Can you work these out from the drawing? Everything is in mm from the part's minimum corner. A direction names the side the tool comes from. Round coordinates to 2 decimals unless told otherwise and drop trailing zeros. Write each loop counter-clockwise with the first axis right and the second up, starting at its lowest first coordinate (ties: lowest second). Pieces come first, ordered by that corner, then holes. Notation, with made-up numbers: (36.5, 27.25) - (46.5, 27.25) arc R17 ccw to (46.5, 54.25) - close; hole circle Ø8 at (11, 66). An arc over 180 degrees is marked (long way). One line per item, written item: value. Start each with the question number.
Item 1: If I drill on line 1 (Y direction, x = 5, z = 16); line 2 (Y direction, x = 4, z = 15); line 3 (Z direction, x = 27.5, y = 13), over which ranges is the centre line in solid material (lowest first)?
Item 2: Imagine slicing it at D-D, the plane y = 16.5. Please give me the cut outline in (x, z), then the cut area to 3 significant figures.
Item 3: Imagine slicing it at B-B, the plane z = 26.67. Please give me the cut outline in (x, y), then the cut area to 3 significant figures.
Item 4: For the marked faces 1 and 2, which set-ups out of +Z, -Z, +X, -X, +Y, -Y let a thin tool reach every point of the face, with its end or its side?
Item 5: For P1, Ø8, axis at x = 20.5, z = 39.5, coming from the +Y side; P2, Ø4, axis at y = 14, z = 27, coming from the -X side, each with a flat end and sliding along its axis, tell me the tip position at first contact or that it passes through.
Item 6: Imagine slicing it at A-A, the plane x = 26.67. Please give me the cut outline in (y, z).
Item 7: Imagine slicing it at C-C, the plane y = 28.5. Please give me the cut outline in (x, z).
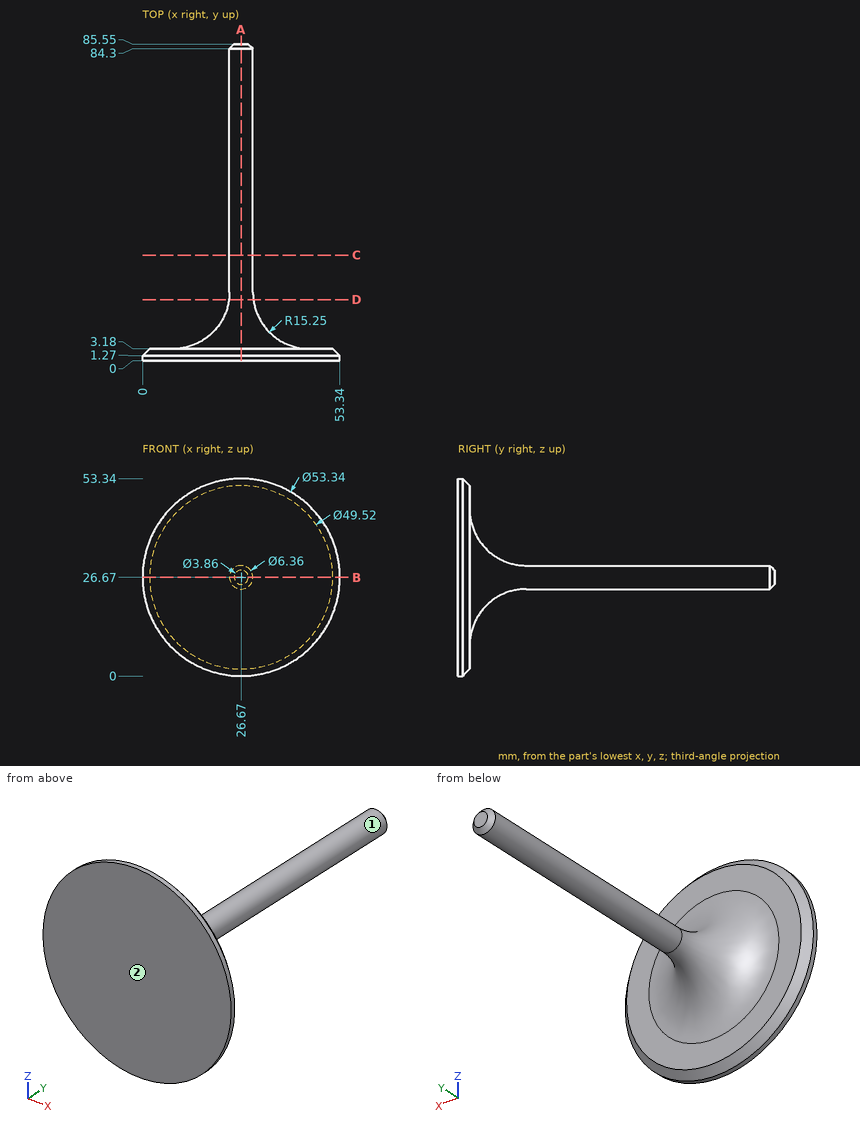
Values follow:
1. line 1: y = 0 to 3.18
1. line 2: y = 0 to 2.44
1. line 3: z = 22.57 to 30.77
2. outline: circle Ø6.61 at (26.67, 26.67)
2. area: 34.3 mm^2
3. outline: (0, 0) - (53.34, 0) - (53.34, 1.27) - (51.43, 3.18) - (45.1, 3.18) arc R15.25 cw to (29.85, 18.43) - (29.85, 84.3) - (28.6, 85.55) - (24.74, 85.55) - (23.49, 84.3) - (23.49, 18.43) arc R15.25 cw to (8.24, 3.18) - (1.91, 3.18) - (0, 1.27) - close
3. area: 788 mm^2
4. face 1: +Y
4. face 2: +Z, -Z, +X, -X, -Y
5. P1: stops at y = 5.57
5. P2: stops at x = 22.07
6. outline: (0, 0) - (1.27, 0) - (3.18, 1.91) - (3.18, 8.24) arc R15.25 cw to (18.43, 23.49) - (84.3, 23.49) - (85.55, 24.74) - (85.55, 28.6) - (84.3, 29.85) - (18.43, 29.85) arc R15.25 cw to (3.18, 45.1) - (3.18, 51.43) - (1.27, 53.34) - (0, 53.34) - close
7. outline: circle Ø6.36 at (26.67, 26.67)
